```python
from build123d import *

# Parameters (mm, degrees)
F0_W     = 254
F0_H     = 177.8
F0_R     = 21.59
F0_R_2   = 25.4
F1_DEPTH = 17.78


with BuildPart() as f1:
    # F0 (on Top) → F1 (new body)
    with BuildSketch(Plane.XY):
        Rectangle(F0_W, F0_H)
        Circle(F0_R, mode=Mode.SUBTRACT)
        with Locations((67.79138, 0)):
            Circle(F0_R_2, mode=Mode.SUBTRACT)
    extrude(amount=F1_DEPTH)


solid = f1.part
```
Build history of the part. All positions in model axes, mm. Round coordinates to 2 decimals unless told otherwise and drop trailing zeros. Loops run counter-clockwise (first coordinate to the right, second up) from the corner with the lowest first, then second, coordinate; pieces in that order, holes last. Notation, with made-up numbers: M 12.5,-32 L 45.5,-32 A19 cw 45.5,0 Z; hole C 30,52 d7. An arc over 180 degrees is marked long. Answer as CSV lines item,"result".
1. Cut at B-B on x = 0. Write the cut outline in (y, z).
Resolved:
outline,"M -88.9,0 L -21.59,0 L -21.59,17.78 L -88.9,17.78 Z; M 21.59,0 L 88.9,0 L 88.9,17.78 L 21.59,17.78 Z"
2. Cut at C-C on z = 8. Write the cut outline in (x, y).
Resolved:
outline,"M -127,-88.9 L 127,-88.9 L 127,88.9 L -127,88.9 Z; hole C 0,0 d43.18; hole C 67.79,0 d50.8"
3. Two-plate mould, pull along Y, no slides. Class faces 1 (the flat face through (-2, -88.9, 9)), 2 (the flat face through (-2, 88.9, 9)), 3 (the cylindrical face through (-15.913, 14.592, 8.766)), 4 (the flat face through (127, -1, 9)): released by +Y, released by -Y, zero draft, split by the parting line, or undercut.
Resolved:
face 1,"released by -Y"
face 2,"released by +Y"
face 3,"undercut"
face 4,"zero draft"
4. Cut at D-D on x = 86.5. Write the cut outline in (y, z).
Resolved:
outline,"M -88.9,0 L -17.18,0 L -17.18,17.78 L -88.9,17.78 Z; M 17.18,0 L 88.9,0 L 88.9,17.78 L 17.18,17.78 Z"
5. Cut at A-A on y = 0. Write the cut outline in (x, z).
Resolved:
outline,"M -127,0 L -21.59,0 L -21.59,17.78 L -127,17.78 Z; M 21.59,0 L 42.39,0 L 42.39,17.78 L 21.59,17.78 Z; M 93.19,0 L 127,0 L 127,17.78 L 93.19,17.78 Z"
6. Wall check: probe 1 along Y at (x, z) = (68.5, 12); probe 2 along X at (y, z) = (11, 2.5); probe 3 along X at (y, z) = (2, 6.25). Give the ranges that are in metal, low to high. Write a range as [from, to].
Resolved:
probe 1,"y = [-88.9, -25.39], [25.39, 88.9]"
probe 2,"x = [-127, -18.58], [18.58, 44.9], [90.69, 127]"
probe 3,"x = [-127, -21.5], [21.5, 42.47], [93.11, 127]"
